CAD build for the part. Positions are in the model's coordinates, mm. A direction names the side the tool comes from. Give positions to 0.01 mm unless a question says otherwise; leave off trailing zeros. Write each loop counter-clockwise with the first axis right and the second up, starting at its lowest first coordinate (ties: lowest second). Pieces come first, ordered by that corner, then holes. Notation, with made-up numbers: M 4.5,65 L 30.5,65 A13 ccw 30.5,90 Z; hole C 62.25,-10 d10. An arc over 180 degrees is marked long. One line per question, with ' | ' between items. Start each with the question number.
1. Cut at A-A, the plane y = 0. Write the cut outline in (x, z).
2. Which spindle directions (+Z, -Z, +X, -X, +Y, -Y) get a long thin tool onto all of the face, cutting with end or side? Do faces 1 (the face through (57.3, -2.818, 31.013)), 2 (the face through (-55, 0, 300)). Say none if no direction does.
3. Cut at B-B, the plane z = 83. Write the cut outline in (x, y).
4. Wall check: L1, parallel to X at y = -1, z = 148.5; L2, parallel to X at y = -1.5, z = 273; L3, parallel to Z at x = 148.5, y = 11.5. Give the ranges that are in metal, low to high.
5. Cut at C-C, the plane x = 47. Write the cut outline in (y, z), then the cut area to 3 significant figures.
6. Flat gauge pins, fed straight in: pin 1 (2 mm diameter, centred on x = 117, y = -4.5, fed in from -Z); pin 2 (6 mm diameter, centred on x = 58, y = -3, fed in from +Z); pin 3 (2 mm diameter, centred on x = -45.5, z = 34, fed in from +Y). Where does each tip first touch, or does it go through?
```python
from build123d import *

# Parameters (mm, degrees)
F0_R     = 17.329579
F1_DEPTH = 300
F3_R     = 13.000421
F4_DEPTH = 200


with BuildPart() as f1:
    # F0 (on Top) → F1 (new body)
    with BuildSketch(Plane.XY):
        with Locations((-54.526214, 0)):
            Circle(F0_R)
    extrude(amount=F1_DEPTH)

    # F3 (on offset) → F4 (join)
    with BuildSketch(Plane.YZ.offset(-41.3)):
        with Locations((0, 43.704636)):
            Circle(F3_R)
    extrude(amount=F4_DEPTH)


solid = f1.part
```
Here are the results:
1) outline: M -71.86,0 L -37.2,0 L -37.2,30.7 L 158.7,30.7 L 158.7,56.71 L -37.2,56.71 L -37.2,300 L -71.86,300 Z
2) face 1: +X | face 2: +Z, +X, -X, +Y, -Y
3) outline: C -54.53,0 d34.66
4) L1: -71.83 to -37.23 | L2: -71.79 to -37.26 | L3: 37.64 to 49.77
5) outline: C 0,43.7 d26 | area: 531 mm^2
6) pin 1: z = 31.18 | pin 2: z = 56.71 | pin 3: y = 15.36
